from build123d import *

# Parameters (mm, degrees)
SKETCH020_R     = 1.75
SKETCH020_R_2   = 2.04611
PAD008_DEPTH    = 5
SKETCH021_R     = 1.75
SKETCH021_R_2   = 1.925729
PAD009_DEPTH    = 1
PAD010_DEPTH    = 47
POCKET010_DEPTH = 1.5
POCKET011_DEPTH = 5
SKETCH025_R     = 1.75
PAD011_DEPTH    = 10
SKETCH026_R     = 3.5
POCKET012_DEPTH = 3.5


with BuildPart() as part:
    # Sketch020 (on Face1 of ShapeBinder) → Pad008 (new body)
    with BuildSketch(Plane.XY.offset(50)):
        with BuildLine():
            ThreePointArc((-51, 69), (-52.414214, 68.414214), (-53, 67))
            Line((-53, -67), (-53, 67))
            ThreePointArc((-53, -67), (-52.414214, -68.414214), (-51, -69))
            Line((51, -69), (-51, -69))
            ThreePointArc((51, -69), (52.414214, -68.414214), (53, -67))
            Line((53, 67), (53, -67))
            ThreePointArc((53, 67), (52.414214, 68.414214), (51, 69))
            Line((-51, 69), (51, 69))
        make_face()
        with Locations((-45, -61)):
            Circle(SKETCH020_R, mode=Mode.SUBTRACT)
        with Locations((45, -61)):
            Circle(SKETCH020_R, mode=Mode.SUBTRACT)
        with Locations((-45, 61)):
            Circle(SKETCH020_R, mode=Mode.SUBTRACT)
        with Locations((45, 61)):
            Circle(SKETCH020_R_2, mode=Mode.SUBTRACT)
    extrude(amount=PAD008_DEPTH)

    # Sketch021 (on Face1 of ShapeBinder) → Pad009 (join)
    with BuildSketch(Plane.XY.offset(50)):
        with BuildLine():
            ThreePointArc((-46.5, 64.5), (-47.914214, 63.914214), (-48.5, 62.5))
            Line((-48.5, -62.5), (-48.5, 62.5))
            ThreePointArc((-48.5, -62.5), (-47.914214, -63.914214), (-46.5, -64.5))
            Line((46.5, -64.5), (-46.5, -64.5))
            ThreePointArc((46.5, -64.5), (47.914214, -63.914214), (48.5, -62.5))
            Line((48.5, 62.5), (48.5, -62.5))
            ThreePointArc((48.5, 62.5), (47.914214, 63.914214), (46.5, 64.5))
            Line((-46.5, 64.5), (46.5, 64.5))
        make_face()
        with Locations((-45, -61)):
            Circle(SKETCH021_R, mode=Mode.SUBTRACT)
        with Locations((45, -61)):
            Circle(SKETCH021_R_2, mode=Mode.SUBTRACT)
        with Locations((-45, 61)):
            Circle(SKETCH021_R, mode=Mode.SUBTRACT)
        with Locations((45, 61)):
            Circle(SKETCH021_R, mode=Mode.SUBTRACT)
    extrude(amount=-PAD009_DEPTH)

    # Sketch022 (on Face14 of Pad008) → Pad010 (join)
    with BuildSketch(Plane.XY.offset(55)):
        with BuildLine():
            Line((3.25, 99), (26.25, 99))
            ThreePointArc((28.25, 97), (27.664214, 98.414214), (26.25, 99))
            Line((28.25, 97), (28.25, 65))
            Line((28.25, 65), (1.25, 65))
            Line((1.25, 65), (1.25, 97))
            ThreePointArc((3.25, 99), (1.835786, 98.414214), (1.25, 97))
        make_face()
    extrude(amount=-PAD010_DEPTH)

    # Sketch023 (on Face30 of Pad010) → Pocket010 (cut)
    with BuildSketch(Plane(origin=(0, 0, 8), x_dir=(1, 0, 0), z_dir=(0, 0, -1))):
        with BuildLine():
            ThreePointArc((7.8, -70), (6.527208, -70.527208), (6, -71.8))
            Line((6, -123.151319), (6, -71.8))
            ThreePointArc((6, -123.151319), (6.527208, -124.424111), (7.8, -124.951319))
            Line((21.8, -124.951319), (7.8, -124.951319))
            ThreePointArc((21.8, -124.951319), (23.072792, -124.424111), (23.6, -123.151319))
            Line((23.6, -71.8), (23.6, -123.151319))
            ThreePointArc((23.6, -71.8), (23.072792, -70.527208), (21.8, -70))
            Line((7.8, -70), (21.8, -70))
        make_face()
        with BuildLine():
            ThreePointArc((10.1, -72.3), (8.827208, -72.827208), (8.3, -74.1))
            Line((8.3, -119.625365), (8.3, -74.1))
            ThreePointArc((8.3, -119.625365), (8.827208, -120.898157), (10.1, -121.425365))
            Line((19.5, -121.425365), (10.1, -121.425365))
            ThreePointArc((19.5, -121.425365), (20.772792, -120.898157), (21.3, -119.625365))
            Line((21.3, -74.1), (21.3, -119.625365))
            ThreePointArc((21.3, -74.1), (20.772792, -72.827208), (19.5, -72.3))
            Line((10.1, -72.3), (19.5, -72.3))
        make_face(mode=Mode.SUBTRACT)
    extrude(amount=-POCKET010_DEPTH, mode=Mode.SUBTRACT)

    # Sketch024 (on Face30 of Pad010) → Pocket011 (cut)
    with BuildSketch(Plane(origin=(0, 0, 8), x_dir=(1, 0, 0), z_dir=(0, 0, -1))):
        Polygon((17.8, -65), (11.8, -65), (11.8, -77.95), (3, -77.95), (3, -82.95), (26.6, -82.95), (26.6, -77.95), (17.8, -77.95), align=None)
    extrude(amount=-POCKET011_DEPTH, mode=Mode.SUBTRACT)

    # Sketch025 (on Face30 of Pad010) → Pad011 (join)
    with BuildSketch(Plane(origin=(0, 0, 8), x_dir=(1, 0, 0), z_dir=(0, 0, -1))):
        with BuildLine():
            Line((-7.75, -73), (-7.75, -80))
            ThreePointArc((-7.75, -80), (-7.457107, -80.707107), (-6.75, -81))
            Line((-6.75, -81), (1.25, -81))
            Line((1.25, -81), (1.25, -72))
            Line((1.25, -72), (-6.75, -72))
            ThreePointArc((-6.75, -72), (-7.457107, -72.292893), (-7.75, -73))
        make_face()
        with Locations((-3.25, -76.5)):
            Circle(SKETCH025_R, mode=Mode.SUBTRACT)
        with BuildLine():
            Line((36.25, -87), (28.25, -87))
            Line((28.25, -87), (28.25, -96))
            Line((28.25, -96), (36.25, -96))
            ThreePointArc((36.25, -96), (36.957107, -95.707107), (37.25, -95))
            Line((37.25, -95), (37.25, -88))
            ThreePointArc((37.25, -88), (36.957107, -87.292893), (36.25, -87))
        make_face()
        with Locations((32.75, -91.5)):
            Circle(SKETCH025_R, mode=Mode.SUBTRACT)
    extrude(amount=-PAD011_DEPTH)

    # Sketch026 (on Face32 of Pad011) → Pocket012 (cut)
    with BuildSketch(Plane.XY.offset(18)):
        with Locations((-3.25, 76.5)):
            Circle(SKETCH026_R)
        with Locations((32.75, 91.5)):
            Circle(SKETCH026_R)
    extrude(amount=-POCKET012_DEPTH, mode=Mode.SUBTRACT)


solid = part.part
Can you work these out from the model? Positions are in its coordinate system, mm. A direction names the side the tool comes from. Give positions to 0.01 mm unless a question says otherwise; leave off trailing zeros. Order: outer loops, then holes, each group sorted by start corner. A loop starts at its lowest first (then second) coordinate and runs counter-clockwise, first axis right, second up. Notation, with made-up numbers: M -4.75,26 L 45.25,26 A22 ccw 45.25,56 Z; hole C 56,86 d2. An arc over 180 degrees is marked long. Use one line per item in the form item = value. Start each with the question number.
Item 1: If I drill on line 1 along Y through (x, z) = (45, 49.6); line 2 along Y through (x, z) = (45, 51); line 3 along Y through (x, z) = (32.75, 16.1), over which ranges is the centre line in solid material (lowest first)?
Item 2: If we section it at B-B (y = -31.5): Write out the boundary of the cut face in (x, z).
Item 3: Will these pins go through, and if not, where does the flat tip stop? pin 1 Ø12 at (x, y) = (-3, 36) entering from -Z; pin 2 Ø3.5 at (x, y) = (33.5, 91.5) entering from +Z; pin 3 Ø2.5 at (x, z) = (-4, 14.5) entering from -Y.
Item 4: We'd pull the mould along Y, two halves only. Please class faces 4 (the flat face through (8, 73, 9.5)), 5 (the flat face through (32, 87, 13)), 6 (the cylindrical face through (31.991, 88.083, 16.274)), 7 (the flat face through (-25, 69, 52)): +Y half, -Y half, draft (parallel to the pull), parting line (faces both ways), or undercut.
Item 5: If we section it at A-A (x = -3.25): Write out the boundary of the cut face in (y, z).
Item 6: For faces 1 (the flat face through (17.8, 72, 10)), 2 (the flat face through (-1, 1, 49)), 3 (the flat face through (-3, 72, 13)), which set-ups out of +Z, -Z, +X, -X, +Y, -Y let a thin tool reach every point of the face, with its end or its side?
Item 7: If we section it at C-C (z = 31): Write out the boundary of the cut face in (x, y), then the cut area to 3 significant figures.
Outcome:
q1.line_1 = -64.5 to -62.93, -59.07 to 59.25, 62.75 to 64.5
q1.line_2 = -69 to -62.75, -59.25 to 58.95, 63.05 to 69
q1.line_3 = 87 to 88, 95 to 96
q2.outline = M -53,50 L -48.5,50 L -48.5,49 L 48.5,49 L 48.5,50 L 53,50 L 53,55 L -53,55 Z
q3.pin_1 = 49
q3.pin_2 = 14.5
q3.pin_3 = 72
q4.face_4 = undercut
q4.face_5 = -Y half
q4.face_6 = undercut
q4.face_7 = +Y half
q5.outline = M -69,50 L -64.5,50 L -64.5,49 L 64.5,49 L 64.5,50 L 69,50 L 69,55 L -69,55 Z; M 72,8 L 74.75,8 L 74.75,14.5 L 73,14.5 L 73,18 L 72,18 Z; M 78.25,8 L 81,8 L 81,18 L 80,18 L 80,14.5 L 78.25,14.5 Z
q6.face_1 = -Z, -Y
q6.face_2 = -Z, +X, -X, -Y
q6.face_3 = +Z, -Z, -X, -Y
q7.outline = M 1.25,65 L 28.25,65 L 28.25,97 A2 ccw 26.25,99 L 3.25,99 A2 ccw 1.25,97 Z
q7.area = 916 mm2
